Check sheet for the modelled part. Datum: model origin and axes. Units: mm. A direction names the side the tool comes from. Give positions to 0.01 mm unless a question says otherwise; leave off trailing zeros. Write each loop counter-clockwise with the first axis right and the second up, starting at its lowest first coordinate (ties: lowest second). Pieces come first, ordered by that corner, then holes. Notation, with made-up numbers: M 53.25,31.25 L 79.25,31.25 A27 cw 79.25,56.25 Z; hole C 32.25,-20.75 d8. An arc over 180 degrees is marked long. Write each question's results on one line, items separated by ' | '. Start each with the question number.
from build123d import *

# Parameters (mm, degrees)
SKETCH_2_R          = 2.3
CUT_EXTRUDE_1_DEPTH = 3.92
CUT_EXTRUDE_START   = -0.62
SKETCH_3_R          = 3.98
SKETCH_3_R_2        = 2.3
CUT_EXTRUDE_2_DEPTH = 0.62


with BuildPart() as part:
    # 草图1 → 旋转1 (revolve)
    with BuildSketch(Plane.XY, mode=Mode.PRIVATE) as revolve_1_sk:
        Polygon((0, 0), (0, 9.64), (2.3, 9.64), (2.3, 5.4), (3.98, 5.4), (3.98, 3.92), (3.12, 3.92), (3.12, 0), align=None)
    revolve(revolve_1_sk.sketch.rotate(Axis((0, 0, 0), (0, 1, 0)), 90), axis=Axis((0, 0, 0), (0, 1, 0)))

    # 草图2 → 切除-拉伸1 (cut)
    with BuildSketch(Plane.XZ):
        with Locations(Location((0, 0, 0), (0, 0, 270))):
            Circle(SKETCH_2_R)
    extrude(amount=-CUT_EXTRUDE_1_DEPTH, mode=Mode.SUBTRACT)

    # 草图3 → 切除-拉伸2 (cut)
    with BuildSketch(Plane(origin=(0, 5.4, 0), x_dir=(1, 0, 0), z_dir=(0, 1, 0)).offset(CUT_EXTRUDE_START)):
        with Locations(Location((0, 0, 0), (0, 0, 90))):
            Circle(SKETCH_3_R)
        with Locations(Location((0, 0, 0), (0, 0, 90))):
            Circle(SKETCH_3_R_2, mode=Mode.SUBTRACT)
    extrude(amount=CUT_EXTRUDE_2_DEPTH, mode=Mode.SUBTRACT)


solid = part.part
Q1. Depth check by flat-ended pin: pin 1 Ø3 at (y, z) = (2, -1.5) entering from +X; pin 2 Ø2 at (x, y) = (-1.5, 7.5) entering from +Z (3 decimals); pin 3 Ø3 at (y, z) = (1.5, 1.5) entering from -X. Enter the tip coordinate at first touch or a pass-through.
Q2. Section check C-C on y = 3.5. Record the boundary of the cut face in (x, z), plus the area to 3 significant figures.
Q3. Release check for a two-part mould opening along X. For faces 4 (the face through (-3.946, 4.344, 0.518)), 5 (the face through (0.691, 1.933, -2.194)), 6 (the face through (0, 3.92, 0)), 7 (the face through (3, 3.92, -2)) record: pulls with the +X half, pulls with the -X half, needs draft (parallel to the pull), parting line crosses it, or undercut.
Q4. Scan lines: L1, parallel to X at y = 1.8, z = 0; L2, parallel to Y at x = -2, z = -1.25; L3, parallel to Y at x = -1, z = -3. Record each from-to range of solid material in increasing order.
Q5. Section check B-B on x = 0. Record the boundary of the cut face in (y, z).
Q6. Section check A-A on z = 0. Record the boundary of the cut face in (x, y).
Q7. Section check D-D on z = -3. Record the boundary of the cut face in (x, y), plus the area to 3 significant figures.
Q8. Tool access check on faces 1 (the face through (0, 9.64, 0)), 2 (the face through (2, 4.78, -2)), 3 (the face through (-0.937, 1.933, -2.976)). Record the directions out of +Z, -Z, +X, -X, +Y, -Y that give a thin tool (end or side, any length) a straight path to the whole face; none if there is none.
Check result:
1) pin 1: x = 3.12 | pin 2: z = 2.245 | pin 3: x = -3.12
2) outline: C 0,0 d6.24; hole C 0,0 d4.6 | area: 14.0 mm^2
3) face 4: parting line crosses it | face 5: undercut | face 6: undercut | face 7: needs draft
4) L1: -3.12 to -2.3, 2.3 to 3.12 | L2: 0 to 4.78 | L3: 3.92 to 4.78
5) outline: M 0,-3.12 L 3.92,-3.12 L 3.92,-3.98 L 4.78,-3.98 L 4.78,-2.3 L 9.64,-2.3 L 9.64,2.3 L 4.78,2.3 L 4.78,3.98 L 3.92,3.98 L 3.92,3.12 L 0,3.12 L 0,2.3 L 3.92,2.3 L 3.92,-2.3 L 0,-2.3 Z
6) outline: M -3.98,3.92 L -3.12,3.92 L -3.12,0 L -2.3,0 L -2.3,3.92 L 2.3,3.92 L 2.3,0 L 3.12,0 L 3.12,3.92 L 3.98,3.92 L 3.98,4.78 L 2.3,4.78 L 2.3,9.64 L -2.3,9.64 L -2.3,4.78 L -3.98,4.78 Z
7) outline: M -2.62,3.92 L -0.86,3.92 L -0.86,0 L 0.86,0 L 0.86,3.92 L 2.62,3.92 L 2.62,4.78 L -2.62,4.78 Z | area: 11.2 mm^2
8) face 1: +Z, -Z, +X, -X, +Y | face 2: +Y | face 3: -Y
